```python
from build123d import *

# Parameters (mm, degrees)
ESQUISSE1_W                                          = 30
ESQUISSE1_H                                          = 60
BOSS_EXTRU_1_DEPTH                                   = 10
ESQUISSE2_W                                          = 30
ESQUISSE2_H                                          = 6
BOSS_EXTRU_2_DEPTH                                   = 70
ESQUISSE3_R                                          = 4
ENL_V_MAT_EXTRU_1_DEPTH                              = 6
ESQUISSE4_W                                          = 30
ESQUISSE4_H                                          = 26.68
BOSS_EXTRU_3_DEPTH                                   = 20
D_GAGEMENT_M31_D                                     = 3.4
D_GAGEMENT_M31_DEPTH                                 = 26.68
D_GAGEMENT_M31_TIP                                   = 1.021463052
CHAMBRAGE_POUR_T_TE_CYLINDRIQUE_FENDUE_M_D           = 3.4
CHAMBRAGE_POUR_T_TE_CYLINDRIQUE_FENDUE_M_DEPTH       = 10
CHAMBRAGE_POUR_T_TE_CYLINDRIQUE_FENDUE_M_CBORE_D     = 6.5
CHAMBRAGE_POUR_T_TE_CYLINDRIQUE_FENDUE_M_CBORE_DEPTH = 2
CHAMBRAGE_POUR_T_TE_CYLINDRIQUE_FENDUE_M_TIP         = 1.021463052
CONG_1_R                                             = 10
ESQUISSE13_W                                         = 6.1
ESQUISSE13_H                                         = 2.4
ENL_V_MAT_EXTRU_2_DEPTH                              = 8.45


with BuildPart() as part:
    # Esquisse1 → Boss.-Extru.1 (new body)
    with BuildSketch(Plane.XY):
        with Locations((15, 30)):
            Rectangle(ESQUISSE1_W, ESQUISSE1_H)
    extrude(amount=BOSS_EXTRU_1_DEPTH)

    # Esquisse2 → Boss.-Extru.2 (add)
    with BuildSketch(Plane.XY.offset(10)):
        with Locations((15, 3)):
            Rectangle(ESQUISSE2_W, ESQUISSE2_H)
    extrude(amount=BOSS_EXTRU_2_DEPTH)

    # Esquisse3 → Enlèv. mat.-Extru.1 (cut)
    with BuildSketch(Plane.XZ):
        with Locations(Location((15, 60, 0), (0, 0, 270))):
            Circle(ESQUISSE3_R)
    extrude(amount=-ENL_V_MAT_EXTRU_1_DEPTH, mode=Mode.SUBTRACT)

    # Esquisse4 → Boss.-Extru.3 (add)
    with BuildSketch(Plane.XY.offset(10)):
        with Locations((15, 46.66)):
            Rectangle(ESQUISSE4_W, ESQUISSE4_H)
    extrude(amount=BOSS_EXTRU_3_DEPTH)

    # Dégagement M31
    with Locations(Plane(origin=(0, 33.32, 0), x_dir=(-1, 0, 0), z_dir=(0, -1, 0))):
        with Locations((-10, -25.25), (-20, -25.25)):
            Hole(D_GAGEMENT_M31_D / 2, depth=D_GAGEMENT_M31_DEPTH)
            with Locations((0, 0, -(D_GAGEMENT_M31_DEPTH + D_GAGEMENT_M31_TIP / 2))):  # 118° drill point
                Cone(0, D_GAGEMENT_M31_D / 2, D_GAGEMENT_M31_TIP, mode=Mode.SUBTRACT)

    # Chambrage pour tête cylindrique fendue M31
    with Locations(Plane.XY.offset(10)):
        with Locations((10, 23.32), (20, 16)):
            CounterBoreHole(CHAMBRAGE_POUR_T_TE_CYLINDRIQUE_FENDUE_M_D / 2, CHAMBRAGE_POUR_T_TE_CYLINDRIQUE_FENDUE_M_CBORE_D / 2, CHAMBRAGE_POUR_T_TE_CYLINDRIQUE_FENDUE_M_CBORE_DEPTH, depth=CHAMBRAGE_POUR_T_TE_CYLINDRIQUE_FENDUE_M_DEPTH)
            with Locations((0, 0, -(CHAMBRAGE_POUR_T_TE_CYLINDRIQUE_FENDUE_M_DEPTH + CHAMBRAGE_POUR_T_TE_CYLINDRIQUE_FENDUE_M_TIP / 2))):  # 118° drill point
                Cone(0, CHAMBRAGE_POUR_T_TE_CYLINDRIQUE_FENDUE_M_D / 2, CHAMBRAGE_POUR_T_TE_CYLINDRIQUE_FENDUE_M_TIP, mode=Mode.SUBTRACT)

    # Congé1
    cong_1_edges = [part.edges().sort_by_distance(p)[0] for p in [
        (30, 3, 80),
        (0, 3, 80),
    ]]
    fillet(cong_1_edges, radius=CONG_1_R)

    # Esquisse13 → Enlèv. mat.-Extru.2 (cut)
    with BuildSketch(Plane.XY.offset(30)):
        with Locations((10, 37.52)):
            Rectangle(ESQUISSE13_W, ESQUISSE13_H)
        with Locations((20, 37.52)):
            Rectangle(ESQUISSE13_W, ESQUISSE13_H)
    extrude(amount=-ENL_V_MAT_EXTRU_2_DEPTH, mode=Mode.SUBTRACT)


solid = part.part
```
CAD build for the part. Positions are in the model's coordinates, mm. A direction names the side the tool comes from. Coordinates: 2 decimals unless noted, no trailing zeros. Write each loop counter-clockwise with the first axis right and the second up, starting at its lowest first coordinate (ties: lowest second). Pieces come first, ordered by that corner, then holes. Notation, with made-up numbers: (-12.5, -36) -> (-3.5, -36) arc R34 ccw to (-3.5, -4) -> close; hole circle Ø2 at (58.25, 69.5). An arc over 180 degrees is marked (long way). Use CSV: the item, a comma, the result in double quotes. Start each with the question number.
Item 1: Drop flat-ended pins along their axis: P1, Ø5, axis at x = 19.5, y = 15, coming from the +Z side; P2, Ø0.7, axis at x = 11, y = 38, coming from the +Z side; P3, Ø5.5, axis at x = 10, y = 23.32, coming from the +Z side; P4, Ø6, axis at y = 10, z = 54.5, coming from the +X side. Give the stop position or say it passes through.
Item 2: Band-saw the part on C-C, the plane x = 15. Write the cut outline in (y, z), plus the area to 3 significant figures.
Item 3: Tool access for faces 1 (the flat face through (30, 34, 17)), 2 (the flat face through (16.95, 38, 26)), 3 (the cylindrical face through (9.779, 49.509, 23.564)), 4 (the flat face through (15, 30, 0)), 5 (the flat face through (15, 20, 10)): list every direction of +Z, -Z, +X, -X, +Y, -Y with a clear straight run to the whole face (end or side of a thin tool).
Item 4: Two-plate mould, pull along Y, no slides. Class faces 6 (the cylindrical face through (20.914, 49.509, 23.817)), 7 (the flat face through (15, 60, 15)), 8 (the flat face through (10, 38, 21.55)): +Y half, -Y half, draft (parallel to the pull), parting line (faces both ways), or undercut.
Item 5: Band-saw the part on B-B, the plane z = 60. Write the cut outline in (x, y), plus the area to 3 significant figures.
Item 6: Band-saw the part on D-D, the plane y = 46. Write the cut outline in (x, z).
Item 7: Wall check: probe 1 along X at (y, z) = (34.9, 25.25); probe 2 along Y at (x, z) = (20, 23.5); probe 3 along X at (y, z) = (23.32, 2.25). Give the ranges that are in metal, low to high.
Item 8: Band-saw the part on A-A, the plane y = 23.32. Write the cut outline in (x, z).
Response values:
1,P1,"stops at z = 10"
1,P2,"stops at z = 21.55"
1,P3,"stops at z = 8"
1,P4,"passes through"
2,outline,"(0, 0) -> (60, 0) -> (60, 30) -> (33.32, 30) -> (33.32, 10) -> (6, 10) -> (6, 56) -> (0, 56) -> close; (0, 64) -> (6, 64) -> (6, 80) -> (0, 80) -> close"
2,area,"1,510 mm2"
3,face 1,"+Z, -Z, +X, +Y, -Y"
3,face 2,"+Z"
3,face 3,"+Y"
3,face 4,"-Z, +X, -X, +Y, -Y"
3,face 5,"+Z, +X, -X"
4,face 6,"draft"
4,face 7,"+Y half"
4,face 8,"undercut"
5,outline,"(0, 0) -> (11, 0) -> (11, 6) -> (0, 6) -> close; (19, 0) -> (30, 0) -> (30, 6) -> (19, 6) -> close"
5,area,"132 mm2"
6,outline,"(0, 0) -> (30, 0) -> (30, 30) -> (0, 30) -> close; hole circle Ø3.4 at (10, 25.25); hole circle Ø3.4 at (20, 25.25)"
7,probe 1,"x = 0 to 8.3, 11.7 to 18.3, 21.7 to 30"
7,probe 2,"y = 0 to 6, 33.32 to 36.32, 38.72 to 60"
7,probe 3,"x = 0 to 8.3, 11.7 to 30"
8,outline,"(0, 0) -> (8.3, 0) -> (8.3, 8) -> (6.75, 8) -> (6.75, 10) -> (0, 10) -> close; (11.7, 0) -> (30, 0) -> (30, 10) -> (13.25, 10) -> (13.25, 8) -> (11.7, 8) -> close"
